Design review of the part built by this model. Coordinates are the model's own, in mm. Face numbers are marked on the shaded views. A direction names the side the tool comes from. Round coordinates to 2 decimals unless told otherwise and drop trailing zeros. Loops run counter-clockwise (first coordinate to the right, second up) from the corner with the lowest first, then second, coordinate; pieces in that order, holes last. Notation, with made-up numbers: M 10,-36 L 29,-36 A5 cw 29,-28 Z; hole C -7,55 d1. An arc over 180 degrees is marked long. Use a Markdown table: item, result.
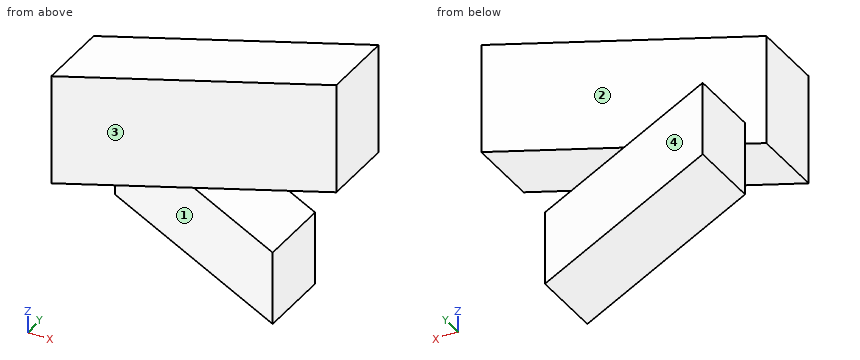
from build123d import *

# Parameters (mm, degrees)
BOSS_EXTRUDE1_DEPTH = 10
BOSS_EXTRUDE3_DEPTH = 15


with BuildPart() as part:
    # Sketch1 → Boss-Extrude1 (new body)
    with BuildSketch(Plane.XY):
        Polygon((-39.908256881, 15.091743119), (-39.908256881, 5.091743119), (-9.908256881, -9.908256881), (-9.908256881, 0.091743119), align=None)
    extrude(amount=BOSS_EXTRUDE1_DEPTH)

    # Sketch2 → Boss-Extrude3 (add)
    with BuildSketch(Plane.XY.offset(10)):
        Polygon((-9.908256881, 15.091743119), (-9.908256881, 5.091743119), (-39.908256881, -9.908256881), (-39.908256881, 0.091743119), align=None)
    extrude(amount=BOSS_EXTRUDE3_DEPTH)


solid = part.part
1. Take a section at C-C on y = 4. Give the boundary of the cut face in (x, z).
Check values:
| item | result |
|---|---|
| outline | M -37.72,0 L -17.72,0 L -17.72,10 L -12.09,10 L -12.09,25 L -32.09,25 L -32.09,10 L -37.72,10 Z |
2. Take a section at D-D on x = -21. Give the boundary of the cut face in (y, z), and give its area (3 significant figures).
Check values:
| item | result |
|---|---|
| outline | M -4.36,0 L 5.64,0 L 5.64,10 L 9.55,10 L 9.55,25 L -0.45,25 L -0.45,10 L -4.36,10 Z |
| area | 250 mm² |
3. Insertion check: pin 1 (10 mm diameter, centred on x = -29.5, y = 11.5, fed in from +Z); pin 2 (1 mm diameter, centred on x = -27, z = 7.5, fed in from +Y); pin 3 (4 mm diameter, centred on x = -33.5, z = 19.5, fed in from -Y). Each pin has a flat end and moves straight along its axis. Give the tip position at first contact, or say it passes through.
Check values:
| item | result |
|---|---|
| pin 1 | stops at z = 10 |
| pin 2 | stops at y = 8.89 |
| pin 3 | stops at y = -7.7 |
4. Machinability: for the marked faces 1, 2, 3 and 4, which of the approach directions +Z, -Z, +X, -X, +Y, -Y give a long, thin tool a straight path to every point of the face, cutting with its end or side? Answer none if there is none.
Check values:
| item | result |
|---|---|
| face 1 | -Z, -X, -Y |
| face 2 | +Z, -X, +Y |
| face 3 | +Z, +X, -Y |
| face 4 | -Z, +X, +Y |
5. Wall thickness on line 1 along Z through (x, y) = (-30.5, -2.5); line 2 along Z through (x, y) = (-33.25, 11.5); line 3 along Y through (x, z) = (-36.75, 16.5): over which ranges is each line inside the solid? List them lowest first. Write a range as from..to.
Check values:
| item | result |
|---|---|
| line 1 | z = 10..25 |
| line 2 | z = 0..10 |
| line 3 | y = -8.33..1.67 |
6. Take a section at A-A on y = -6.25. Give the boundary of the cut face in (x, z).
Check values:
| item | result |
|---|---|
| outline | M -39.91,10 L -32.59,10 L -32.59,25 L -39.91,25 Z; M -17.22,0 L -9.91,0 L -9.91,10 L -17.22,10 Z |
7. Take a section at B-B on x = -14.25. Give the boundary of the cut face in (y, z), and give its area (3 significant figures).
Check values:
| item | result |
|---|---|
| outline | M -7.74,0 L 2.26,0 L 2.26,10 L -7.74,10 Z; M 2.92,10 L 12.92,10 L 12.92,25 L 2.92,25 Z |
| area | 250 mm² |
